Design review of the part built by this model. Coordinates are the model's own, in mm. A direction names the side the tool comes from. Coordinates: 2 decimals unless noted, no trailing zeros. Order: outer loops, then holes, each group sorted by start corner. A loop starts at its lowest first (then second) coordinate and runs counter-clockwise, first axis right, second up. Notation, with made-up numbers: (27, 5) -> (83, 5) arc R24 ccw to (83, 19) -> close; hole circle Ø8 at (18, 38.5). An arc over 180 degrees is marked (long way). Use a Markdown table: item, result. Add a question column.
Q1. Add section B-B (z = -38.5). State the section outline as (x, y) points, then the cut area to 3 significant figures.
Q2. Insertion check: pin 1 (4 mm diameter, centred on x = 111.5, y = 8.5, fed in from -Z); pin 2 (2 mm diameter, centred on y = 3, z = -20.5, fed in from -X); pin 3 (6 mm diameter, centred on y = 8, z = -6, fed in from -X). Each pin has a flat end and moves straight along its axis. Give the tip position at first contact, or say it passes through.
Q3. Machinability: for faces 1 (the face through (153.2, 6.26, -24.24)), 2 (the face through (63, 6, 0)), which of the approach directions +Z, -Z, +X, -X, +Y, -Y give a long, thin tool a straight path to every point of the face, cutting with its end or side? Answer none if there is none.
Q4. Add section D-D (x = 3.5). State the section outline as (y, z) points, then the cut area to 3 significant figures.
Q5. The part is to be moulded in two halves that separate along X. For faces 3 (the face through (-24.1, 6.3, -20.7)), 4 (the face through (70, 12.7, 1)), 5 (the face through (150.662, 6.261, -23.147)), 6 (the face through (-26.428, 6.261, -19.264)), say which applies: pulls with the +X half, pulls with the -X half, needs draft (parallel to the pull), parting line crosses it, or undercut.
Q6. Wall thickness on probe 1 along X at (y, z) = (8.25, -24.5); probe 2 along Z at (x, y) = (64.5, 1.75); probe 3 along X at (y, z) = (7.25, -3.5): over which ranges is each line inside the solid? List them lowest first.
Q7. Add section A-A (y = 8.5). State the section outline as (x, z) points, then the cut area to 3 significant figures.
Q8. Add section C-C (z = -20.5). State the section outline as (x, y) points.
from build123d import *

# Parameters (mm, degrees)
EXTRUDE_THIN1_DEPTH = 12.7


with BuildPart() as part:
    # Sketch1 → Extrude-Thin1 (new body)
    with BuildSketch(Plane(origin=(0, 0, 0), x_dir=(1, 0, 0), z_dir=(0, 1, 0))):
        with BuildLine():
            ThreePointArc((-8.201608063, 47.335515762), (-24.020394602, 20.216381636), (0, 0))
            Line((0, 0), (127, 0))
            ThreePointArc((127, 0), (150.667757881, 23.667757881), (127, 47.335515762))
            Line((127, 47.335515762), (127, 49.875515762))
            ThreePointArc((127, 49.875515762), (153.207757881, 23.667757881), (127, -2.54))
            Line((127, -2.54), (0, -2.54))
            ThreePointArc((0, -2.54), (-26.52310557, 19.782748367), (-9.056142503, 49.727454493))
            Line((-9.056142503, 49.727454493), (-8.201608063, 47.335515762))
        make_face()
    extrude(amount=EXTRUDE_THIN1_DEPTH)


solid = part.part
Established:
| question | item | result |
|---|---|---|
| 1 | outline | (-22.92, 0) -> (-19.87, 0) -> (-19.87, 12.7) -> (-22.92, 12.7) -> close; (145.44, 0) -> (148.61, 0) -> (148.61, 12.7) -> (145.44, 12.7) -> close |
| 1 | area | 78.8 mm^2 |
| 2 | pin 1 | z = 0 |
| 2 | pin 2 | x = -26.76 |
| 2 | pin 3 | x = -22.09 |
| 3 | face 1 | +X, +Y, -Y |
| 3 | face 2 | -Z, +Y, -Y |
| 4 | outline | (0, 0) -> (12.7, 0) -> (12.7, 2.54) -> (0, 2.54) -> close |
| 4 | area | 32.3 mm^2 |
| 5 | face 3 | undercut |
| 5 | face 4 | needs draft |
| 5 | face 5 | undercut |
| 5 | face 6 | pulls with the -X half |
| 6 | probe 1 | -26.92 to -24.38, 150.65 to 153.19 |
| 6 | probe 2 | 0 to 2.54 |
| 6 | probe 3 | -16.99 to -12.59, 139.39 to 143.74 |
| 7 | outline | (-9.06, -49.73) -> (-8.2, -47.34) arc R24.38 cw to (0, 0) -> (127, 0) arc R23.67 cw to (127, -47.34) -> (127, -49.88) arc R26.21 ccw to (127, 2.54) -> (0, 2.54) arc R26.92 ccw to start |
| 7 | area | 704 mm^2 |
| 8 | outline | (-26.64, 0) -> (-24.07, 0) -> (-24.07, 12.7) -> (-26.64, 12.7) -> close; (150.45, 0) -> (153.02, 0) -> (153.02, 12.7) -> (150.45, 12.7) -> close |
